Build history of the part. All positions in model axes, mm. A direction names the side the tool comes from. Coordinates: 2 decimals unless noted, no trailing zeros. Order: outer loops, then holes, each group sorted by start corner. A loop starts at its lowest first (then second) coordinate and runs counter-clockwise, first axis right, second up. Notation, with made-up numbers: (55, 12.25) - (97, 12.25) arc R26 ccw to (97, 43.25) - close; hole circle Ø11 at (12.25, 65). An arc over 180 degrees is marked (long way). Write each question's results on one line, items separated by ' | '.
from build123d import *

# Parameters (mm, degrees)
PAD015_DEPTH         = 350
POCKET024_DEPTH      = 2.001
POCKET024_DEPTH_BACK = 20.001
PAD016_DEPTH         = 20
SKETCH051_R          = 1.5
POCKET029_DEPTH      = 5
SKETCH052_R          = 1.5
POCKET030_DEPTH      = 5
SKETCH053_R          = 1.5
POCKET031_DEPTH      = 5
SKETCH054_R          = 1.5
POCKET032_DEPTH      = 5
SKETCH055_R          = 1.5
POCKET033_DEPTH      = 5
SKETCH065_R          = 1.5
POCKET041_DEPTH      = 24.001


with BuildPart() as part:
    # Sketch044 (on Face1 of Binder013) → Pad015 (new body)
    with BuildSketch(Plane(origin=(0, -0.1, 0), x_dir=(-1, 0, 0), z_dir=(0, 1, 0))):
        Polygon((100, -343.2), (100, -341.2), (120, -341.2), (120, 122.9396985174), (100, 124.9073888451), (100, 126.9073888451), (122, 124.9396985174), (122, -343.2), align=None)
    extrude(amount=PAD015_DEPTH)

    # Sketch045 (on Face3 of Pad015) → Pocket024 (cut, two sides)
    with BuildSketch(Plane.YZ.offset(-120)) as pocket024_sk:
        Polygon((-0.1, -203.2), (190.4875899006, 126.907389), (-0.1, 126.907389), align=None)
    extrude(amount=-POCKET024_DEPTH, mode=Mode.SUBTRACT)
    extrude(pocket024_sk.sketch, amount=POCKET024_DEPTH_BACK, mode=Mode.SUBTRACT)

    # Sketch046 (on Face7 of Pocket024) → Pad016 (join)
    with BuildSketch(Plane.YZ.offset(-120)):
        Polygon((188.1968427325, 122.9396985174), (190.1968427325, 122.9396985174), (1.9, -203.2), (1.9, -341.2), (-0.1, -341.2), (-0.1, -203.2), align=None)
    extrude(amount=PAD016_DEPTH)

    # Sketch051 (on Face14 of Pad016) → Pocket029 (cut)
    with BuildSketch(Plane(origin=(0, 87.9131810245, -50.7566987298), x_dir=(1, 0, 0), z_dir=(0, -0.8660254038, 0.5))):
        with Locations((-110, 190.567323)):
            Circle(SKETCH051_R)
        with Locations((-110, 106.418902)):
            Circle(SKETCH051_R)
        with Locations((-110, 12.270481)):
            Circle(SKETCH051_R)
        with Locations((-110, -76.877941)):
            Circle(SKETCH051_R)
        with Locations((-110, -166.026362)):
            Circle(SKETCH051_R)
    extrude(amount=-POCKET029_DEPTH, mode=Mode.SUBTRACT)

    # Sketch052 (on Face14 of Pocket029) → Pocket030 (cut)
    with BuildSketch(Plane.XZ.offset(0.1)):
        with Locations((-110, -333.2)):
            Circle(SKETCH052_R)
        with Locations((-110, -273.2)):
            Circle(SKETCH052_R)
        with Locations((-110, -213.2)):
            Circle(SKETCH052_R)
    extrude(amount=-POCKET030_DEPTH, mode=Mode.SUBTRACT)

    # Sketch053 (on Face1 of Pocket030) → Pocket031 (cut)
    with BuildSketch(Plane.XY.offset(-341.2)):
        with Locations((-110, 339.9)):
            Circle(SKETCH053_R)
        with Locations((-110, 175.9)):
            Circle(SKETCH053_R)
        with Locations((-110, 93.9)):
            Circle(SKETCH053_R)
        with Locations((-110, 11.9)):
            Circle(SKETCH053_R)
        with Locations((-110, 257.9)):
            Circle(SKETCH053_R)
    extrude(amount=-POCKET031_DEPTH, mode=Mode.SUBTRACT)

    # Sketch054 (on Face21 of Pocket031) → Pocket032 (cut)
    with BuildSketch(Plane(origin=(-12.0541875412, 0, 134.7733035964), x_dir=(0.9960240399, 0, 0.0890848577), z_dir=(-0.0890848577, 0, 0.9960240399))):
        with Locations((-98.296877, 200.48759)):
            Circle(SKETCH054_R)
        with Locations((-98.296877, 270.193795)):
            Circle(SKETCH054_R)
        with Locations((-98.296877, 339.9)):
            Circle(SKETCH054_R)
    extrude(amount=-POCKET032_DEPTH, mode=Mode.SUBTRACT)

    # Sketch055 (on Face21 of Pocket031) → Pocket033 (cut)
    with BuildSketch(Plane(origin=(-12.0541875412, 0, 134.7733035964), x_dir=(0.9960240399, 0, 0.0890848577), z_dir=(-0.0890848577, 0, 0.9960240399))):
        with Locations((-98.296877, 200.48759)):
            Circle(SKETCH055_R)
        with Locations((-98.296877, 339.9)):
            Circle(SKETCH055_R)
        with Locations((-98.296877, 270.193795)):
            Circle(SKETCH055_R)
    extrude(amount=-POCKET033_DEPTH, mode=Mode.SUBTRACT)

    # Sketch065 (on Face1 of Binder018) → Pocket041 (cut, through all)
    with BuildSketch(Plane(origin=(-124, 0, 0), x_dir=(0, -1, 0), z_dir=(-1, 0, 0))):
        with Locations((-339.9, -213.2)):
            Circle(SKETCH065_R)
        with Locations((-257.9, -213.2)):
            Circle(SKETCH065_R)
        with Locations((-175.9, -213.2)):
            Circle(SKETCH065_R)
        with Locations((-93.9, -213.2)):
            Circle(SKETCH065_R)
        with Locations((-11.9, -213.2)):
            Circle(SKETCH065_R)
    extrude(amount=-POCKET041_DEPTH, mode=Mode.SUBTRACT)


solid = part.part
1. Tool access for faces 4 (the face through (-122, 211, -158)), 5 (the face through (-110, 173, -341.2)): list every direction of +Z, -Z, +X, -X, +Y, -Y with a clear straight run to the whole face (end or side of a thin tool).
Solved:
face 4: +Z, -Z, -X, +Y, -Y | face 5: +X, +Y
2. Band-saw the part on B-B on y = 307. Give the cut face in (x, z).
Solved:
outline: (-122, -343.2) - (-100, -343.2) - (-100, -341.2) - (-120, -341.2) - (-120, 122.94) - (-100, 124.91) - (-100, 126.91) - (-122, 124.94) - close
3. Two-plate mould, pull along Z, no slides. Class faces 1 (the face through (-120, 212, -164)), 2 (the face through (-114, -0.1, -274)), 3 (the face through (-113.6, 93.86, -40.46)): +Z half, -Z half, draft (parallel to the pull), parting line (faces both ways), or undercut.
Solved:
face 1: undercut | face 2: draft | face 3: +Z half
4. Drop flat-ended pins along their axis: pin 1 Ø4 at (x, z) = (-108.5, -12) entering from +Y; pin 2 Ø2.5 at (y, z) = (11.9, -213.2) entering from +X; pin 3 Ø5 at (x, y) = (-111, 128.5) entering from +Z; pin 4 Ø3 at (x, y) = (-111.5, 66.5) entering from +Z. Give the stop position or say it passes through.
Solved:
pin 1: stops at y = 113.44 | pin 2: passes through | pin 3: stops at z = 23.87 | pin 4: stops at z = -85.25
5. Band-saw the part on A-A on x = -104. Give the cut face in (y, z).
Solved:
outline: (-0.1, -343.2) - (349.9, -343.2) - (349.9, -341.2) - (1.9, -341.2) - (1.9, -203.2) - (190.2, 122.94) - (188.2, 122.94) - (-0.1, -203.2) - close; (189.11, 124.51) - (349.9, 124.51) - (349.9, 126.55) - (190.28, 126.55) - close
6. Probe line 1 (Y direction, x = -120.4, z = -213.2); line 2 (Z direction, x = -110, y = 1.35); line 3 (X direction, y = 298.5, z = -100). List the from-to ranges inside material, lowest first.
Solved:
line 1: y = -0.1 to 10.4, 13.4 to 92.4, 95.4 to 174.4, 177.4 to 256.4, 259.4 to 338.4, 341.4 to 349.9 | line 2: z = -343.2 to -334.7, -331.7 to -274.7, -271.7 to -214.7, -211.7 to -200.69 | line 3: x = -122 to -120
7. Band-saw the part on C-C on z = -287.5. Give the cut face in (x, y), then the cut area to 3 significant figures.
Solved:
outline: (-122, -0.1) - (-100, -0.1) - (-100, 1.9) - (-120, 1.9) - (-120, 349.9) - (-122, 349.9) - close | area: 740 mm2
8. Band-saw the part on D-D on y = 159.5. Give the cut face in (x, z).
Solved:
outline: (-122, -343.2) - (-100, -343.2) - (-100, -341.2) - (-120, -341.2) - (-120, 69.77) - (-100, 69.77) - (-100, 73.24) - (-122, 73.24) - close
